Read the model definition and answer for the solid it produces. Units are mm, in the model's axes. Face numbers are marked on the shaded views. A direction names the side the tool comes from. Coordinates: 2 decimals unless noted, no trailing zeros. Write each loop counter-clockwise with the first axis right and the second up, starting at its lowest first coordinate (ties: lowest second). Pieces come first, ordered by that corner, then holes.
Item 1: A tool of negligible diameter and unlimited length cuts with its end or side. For the marked faces 4, 5, 6 and 7, from which of +Z, -Z, +X, -X, +Y, -Y can it reach the whole face along a straight path? Write none if from no direction.
Item 2: Determine the mould class of the marked faces 1, 2 and 3 for opening direction Y: released by +Y, released by -Y, zero draft, split by the parting line, or undercut.
Item 3: Straight lines are drawn through the part: probe 1 along Y at (x, z) = (-5, 0.55); probe 2 along Y at (x, z) = (-3.25, 0.9); probe 3 along Y at (x, z) = (-5.5, 1.2). For each, find the intervals that lie inside material, in ascending order.
Item 4: Section C-C (y = 11.5) is taken. Give the vertices of the cut face in (x, z), then the cut area to 3 significant figures.
Item 5: Section D-D (y = 18) is taken. Give the vertices of the cut face in (x, z).
Item 6: Section A-A (y = 9.5) is taken. Give the vertices of the cut face in (x, z), then the cut area to 3 significant figures.
Item 7: Each of these flat-tipped pins is pushed along its axis until it touches: P1, Ø0.8, axis at y = 15.5, z = 0.5, coming from the -X side; P2, Ø4, axis at x = -5.5, y = 16.5, coming from the +Z side; P3, Ø0.5, axis at x = -8.5, z = 0.5, coming from the +Y side; P4, Ø3, axis at x = -3, y = 9.5, coming from the -Z side. Where does it stop, or does it pass through?
Autodesk Inventor part; units mm, degrees
ref_plane "YZ Plane" through (0, 0, 0) normal (1, 0, 0) x (0, 1, 0)
ref_plane "XZ Plane" through (0, 0, 0) normal (0, 1, 0) x (-1, 0, 0)
ref_plane "XY Plane" through (0, 0, 0) normal (0, 0, 1) x (1, 0, 0)
sketch "Boceto1" plane through (0, 0, 0) normal (0, 0, 1) x (1, 0, 0)
  circle A0 centre (-5, 18) radius 1
  line L0 (-8.3939, 13.4965) -> (-8, 13)
  line L1 (-8, 13) -> (-8, 12)
  line L2 (-2, 13) -> (-2, 12)
  line L3 (-2, 13) -> (-1.6061, 13.4965)
  line L4 (-1.6061, 13.4965) -> (-1.8061, 13.4965)
  line L5 (-1.8061, 13.4965) -> (-2.2146, 13.1547)
  line L6 (-2.2146, 13.1547) -> (-2.2146, 14.1547)
  line L7 (-2.2146, 14.1547) -> (-2.5, 14.1547)
  line L8 (-2.5, 14.1547) -> (-2.5, 19.2702)
  line L9 (-2.5, 19.2702) -> (-2.9213, 20)
  line L10 (-2.9213, 20) -> (-7.0787, 20)
  line L11 (-7.0787, 20) -> (-7.5, 19.2702)
  line L12 (-7.5, 19.2702) -> (-7.5, 14.1547)
  line L13 (-7.5, 14.1547) -> (-7.7854, 14.1547)
  line L14 (-7.7854, 14.1547) -> (-7.7854, 13.1547)
  line L15 (-7.7854, 13.1547) -> (-8.1939, 13.4965)
  line L16 (-8.1939, 13.4965) -> (-8.3939, 13.4965)
  line L17 (-8, 12) -> (-9, 12)
  line L18 (-9, 12) -> (-9, 8)
  line L19 (-7, 8) -> (-9, 8)
  line L20 (-7, 8) -> (-7, 11)
  line L21 (-3, 11) -> (-3, 8)
  line L22 (-1, 8) -> (-3, 8)
  line L23 (-1, 12) -> (-1, 8)
  line L24 (-1, 12) -> (-2, 12)
  line L25 (-3, 11) -> (-7, 11)
  point P0 (0, 0)
extrude "Extrusión1" add sketch "Boceto1" along normal blind 1
sketch "Boceto8" plane through (0, 0, 1) normal (0, 0, 1) x (1, 0, 0)
  line L0 (-3.001, 11.0119) -> (-7.001, 11.0119)
  line L1 (-7.001, 11.0119) -> (-7.001, 12.0119)
  line L2 (-7.001, 12.0119) -> (-3.001, 12.0119)
  line L3 (-3.001, 12.0119) -> (-3.001, 11.0119)
  point P0 (0, 0)
  dimension "d24" = 4
  dimension "d25" = 1
extrude "Extrusión4" add sketch "Boceto8" along normal blind 3
fillet "Empalme5" radius 0.7 2 edges at (-7.001, 11.5119, 4) (-3.001, 11.5119, 4)
properties material "----------"
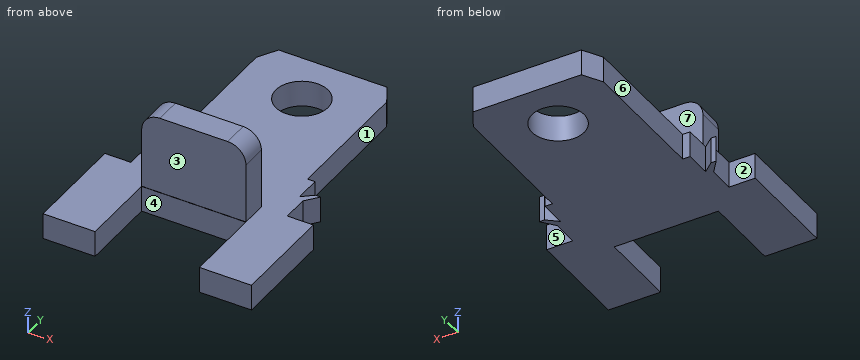
Established:
1. face 4: +Z, -Z, -Y
1. face 5: +Z, -Z, +X
1. face 6: +Z, -Z, -X, +Y
1. face 7: +Z, +X, -X, +Y
2. face 1: zero draft
2. face 2: undercut
2. face 3: released by -Y
3. probe 1: y = 11 to 17, 19 to 20
3. probe 2: y = 11 to 20
3. probe 3: y = 11.01 to 12.01
4. outline: (-9, 0) - (-1, 0) - (-1, 1) - (-3, 1) - (-3, 3.3) arc R0.7 ccw to (-3.7, 4) - (-6.3, 4) arc R0.7 ccw to (-7, 3.3) - (-7, 1) - (-9, 1) - close
4. area: 19.8 mm2
5. outline: (-7.5, 0) - (-6, 0) - (-6, 1) - (-7.5, 1) - close; (-4, 0) - (-2.5, 0) - (-2.5, 1) - (-4, 1) - close
6. outline: (-9, 0) - (-7, 0) - (-7, 1) - (-9, 1) - close; (-3, 0) - (-1, 0) - (-1, 1) - (-3, 1) - close
6. area: 4.00 mm2
7. P1: stops at x = -7.5
7. P2: stops at z = 1
7. P3: stops at y = 13.5
7. P4: stops at z = 0
